For this review, use the dimensioned drawing (mm, ordinates from the lowest corner) and the shaded views. A direction names the side the tool comes from. Give positions to 0.01 mm unless a question says otherwise; leave off trailing zeros. Write each loop counter-clockwise with the first axis right and the second up, starting at its lowest first coordinate (ties: lowest second). Pieces come first, ordered by that corner, then holes.
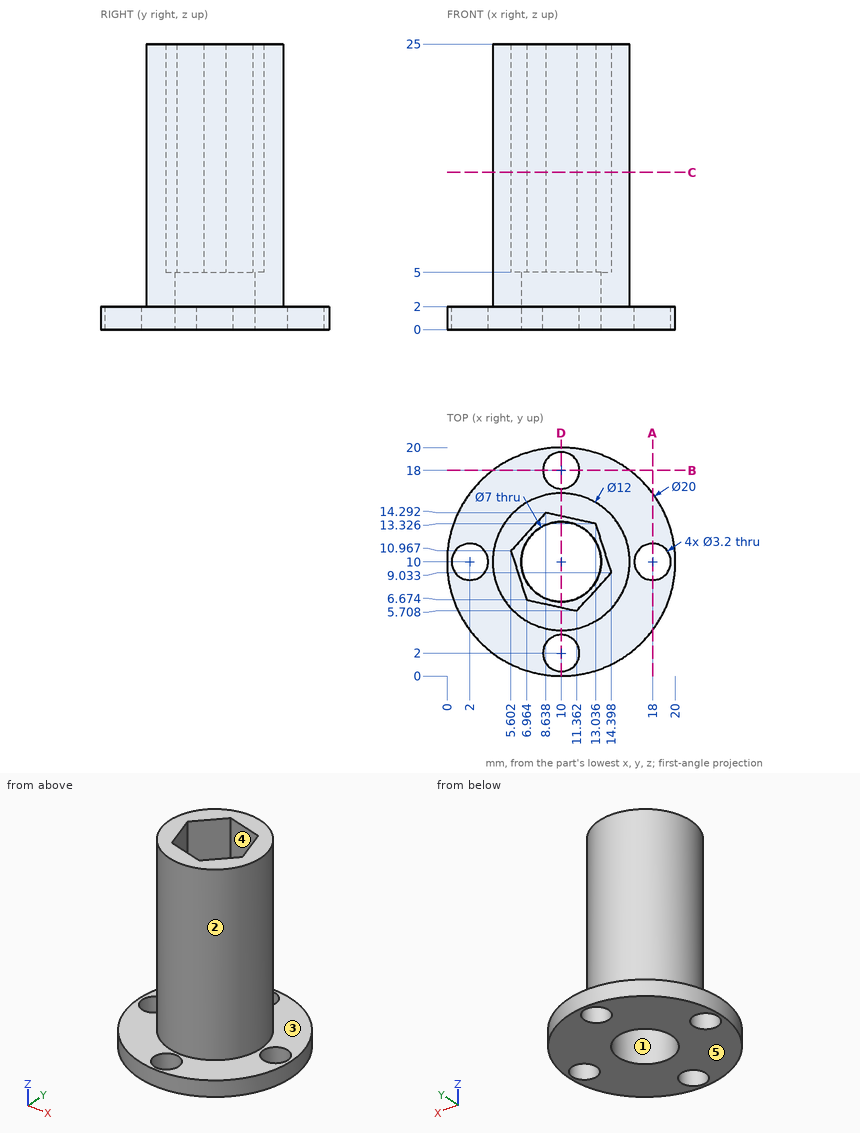
(1) We need section A-A (x = 18). Write out the cut boundary in (y, z), and give its area (3 significant figures).
(2) We need section D-D (x = 10). Write out the cut boundary in (y, z).
(3) We need section C-C (z = 13.75). Write out the cut boundary in (x, y) (1 decimal).
(4) Tool access review of the marked faces 4 and 5: name each direction out of +Z, -Z, +X, -X, +Y, -Y from which nothing blocks a thin tool from reaching the whole face with its end or side.
(5) The part is to be moulded in two halves that separate along Y. For the marked faces 1, 2 and 3, say which applies: +Y half, -Y half, draft (parallel to the pull), parting line (faces both ways), or undercut.
(6) For L1, parallel to X at y = 18, z = 1.15; L2, parallel to Y at x = 7, z = 11.75 (1 decimal), list the stretches that pass through material, from the lowest coordinate up.
(7) Clearance check with flat-ended pins moving along their axes: pin 1 Ø5 at (x, z) = (11.5, 12) entering from -Y; pin 2 Ø12 at (x, z) = (3.5, 3.5) entering from -Y; pin 3 Ø6 at (y, z) = (4.5, 11.5) entering from -X (1 decimal). State where each tip first meets the part, or that it passes through.
The answers:
1. outline: (4, 0) - (8.4, 0) - (8.4, 2) - (4, 2) - close; (11.6, 0) - (16, 0) - (16, 2) - (11.6, 2) - close
1. area: 17.6 mm2
2. outline: (0, 0) - (0.4, 0) - (0.4, 2) - (0, 2) - close; (3.6, 0) - (6.5, 0) - (6.5, 5) - (6.01, 5) - (6.01, 25) - (4, 25) - (4, 2) - (3.6, 2) - close; (13.5, 0) - (16.4, 0) - (16.4, 2) - (16, 2) - (16, 25) - (13.99, 25) - (13.99, 5) - (13.5, 5) - close; (19.6, 0) - (20, 0) - (20, 2) - (19.6, 2) - close
3. outline: circle Ø12 at (10, 10); hole (5.6, 11) - (7, 6.7) - (11.4, 5.7) - (14.4, 9) - (13, 13.3) - (8.6, 14.3) - close
4. face 4: +Z
4. face 5: -Z, +X, -X, +Y, -Y
5. face 1: undercut
5. face 2: parting line
5. face 3: draft
6. L1: x = 4 to 8.4, 11.6 to 16
6. L2: y = 4.8 to 6.7, 12.5 to 15.2
7. pin 1: stops at y = 4
7. pin 2: stops at y = 0.02
7. pin 3: stops at x = 4.5
